Autodesk Fusion 360 part; units mm, degrees
sketch "Sketch1" plane through (0, 0, 0) normal (0, 1, 0) x (1, 0, 0)
  line L0 (0, 0) -> (60, 0)
  line L1 (60, 0) -> (-60, 0)
  line L2 (-60, 0) -> (-60, -50)
  line L3 (-60, -50) -> (60, -50)
  line L4 (60, -50) -> (60, 0)
  line L5 (-60, 0) -> (-45, 0)
  line L6 (60, 0) -> (45, 0)
  line L7 (-45, 0) -> (-45, 60)
  line L8 (45, 0) -> (45, 60)
  line L9 (-45, 60) -> (45, 60)
  dimension "d1" = 60
  dimension "d2" = 120
  dimension "d3" = 50
  dimension "d4" = 15
  dimension "d5" = 15
  dimension "d6" = 60
  dimension "d7" = 60
extrude "Extrude1" add sketch "Sketch1" along normal blind 10
sketch "Sketch2" plane through (0, 10, 0) normal (0, 1, 0) x (-1, 0, 0)
  line L0 (60, 0) -> (60, 50)
  line L1 (60, 50) -> (-60, 50)
  line L2 (-60, 50) -> (-60, 0)
  line L3 (-60, 0) -> (-45, 0)
  line L4 (-45, 0) -> (-45, -60)
  line L5 (-45, -60) -> (45, -60)
  line L6 (45, -60) -> (45, 0)
  line L7 (45, 0) -> (60, 0)
  line L8 (60, 50) -> (60, 40)
  line L9 (-60, 50) -> (-60, 40)
  circle A0 centre (50, 40) radius 2.5
  circle A1 centre (-50, 40) radius 2.5
  circle A2 centre (50, 10) radius 2.5
  circle A3 centre (-50, 10) radius 2.5
  dimension "d10" = 10
  dimension "d11" = 10
  dimension "d12" = 10
  dimension "d13" = 10
  dimension "d14" = 5
  dimension "d15" = 5
  dimension "d16" = 30
  dimension "d17" = 5
  dimension "d18" = 30
  dimension "d19" = 5
extrude "Extrude2" cut sketch "Sketch2" against normal blind 20 contours A0 | A1 | A2 | A3
sketch "Sketch3" plane through (0, 10, 0) normal (0, 1, 0) x (-1, 0, 0)
  circle A0 centre (50, 40) radius 2.5
  circle A1 centre (-50, 40) radius 2.5
  circle A2 centre (50, 10) radius 2.5
  circle A3 centre (-50, 10) radius 2.5
  line L0 (60, 0) -> (60, 50)
  line L1 (60, 50) -> (-60, 50)
  line L2 (-60, 50) -> (-60, 0)
  line L3 (-60, 0) -> (-45, 0)
  line L4 (-45, 0) -> (-45, -60)
  line L5 (-45, -60) -> (45, -60)
  line L6 (45, -60) -> (45, 0)
  line L7 (45, 0) -> (60, 0)
  line L8 (45, -60) -> (45, 50)
  line L9 (-45, -60) -> (-45, 50)
  line L10 (45, 50) -> (-45, 50)
  line L11 (-45, -60) -> (45, -60)
  line L12 (45, 50) -> (42, 50)
  line L13 (45, -60) -> (42, -60)
  line L14 (-45, -60) -> (-45, -57)
  line L15 (-45, 50) -> (-42, 50)
  line L16 (42, 47) -> (42, -57)
  line L17 (-42, -57) -> (42, -57)
  line L18 (-42, -57) -> (-42, 47)
  line L19 (-42, 47) -> (42, 47)
  dimension "d22" = 3
  dimension "d23" = 3
  dimension "d24" = 3
  dimension "d25" = 3
  dimension "d26" = 3
  dimension "d27" = 3
  dimension "d28" = 3
  dimension "d29" = 3
extrude "Extrude3" add sketch "Sketch3" along normal blind 70 contours L1 L4 L5 L6 L8 L9 L10 L11 L12 L13 L14 L15
sketch "Sketch4" plane through (-45, 0, 0) normal (-1, 0, 0) x (0, 0, 1)
  line L0 (-60, 0) -> (0, 0)
  line L1 (0, 0) -> (0, 10)
  line L2 (0, 10) -> (50, 10)
  line L3 (50, 10) -> (50, 80)
  line L4 (50, 80) -> (-60, 80)
  line L5 (-60, 80) -> (-60, 0)
  line L6 (-60, 80) -> (-60, 75)
  circle A0 centre (-35, 75) radius 2.5
  circle A1 centre (25, 75) radius 2.5
  dimension "d32" = 25
  dimension "d34" = 5
  dimension "d35" = 5
extrude "Extrude4" cut sketch "Sketch4" against normal blind 10 contours A0 | A1
sketch "Sketch5" plane through (45, 0, 0) normal (1, 0, 0) x (0, 0, -1)
  line L0 (0, 0) -> (60, 0)
  line L1 (60, 0) -> (60, 80)
  line L2 (60, 80) -> (-50, 80)
  line L3 (-50, 80) -> (-50, 10)
  line L4 (-50, 10) -> (0, 10)
  line L5 (0, 10) -> (0, 0)
  line L6 (-50, 80) -> (-50, 75)
  circle A0 centre (-25, 75) radius 2.5
  circle A1 centre (35, 75) radius 2.5
  dimension "d38" = 5
  dimension "d39" = 25
  dimension "d41" = 5
  dimension "d42" = 5
extrude "Extrude5" cut sketch "Sketch5" against normal blind 11 contours A0 | A1
sketch "Sketch6" plane through (0, 0, 50) normal (0, 0, 1) x (1, 0, 0)
  line L0 (-60, 0) -> (60, 0)
  line L1 (60, 0) -> (60, 10)
  line L2 (60, 10) -> (45, 10)
  line L3 (45, 10) -> (45, 80)
  line L4 (45, 80) -> (-45, 80)
  line L5 (-45, 80) -> (-45, 10)
  line L6 (-45, 10) -> (-60, 10)
  line L7 (-60, 10) -> (-60, 0)
  circle A0 centre (0, 75) radius 2.5
  dimension "d47" = 5
extrude "Extrude6" cut sketch "Sketch6" against normal blind 11 contours A0
sketch "Sketch7" plane through (0, 0, -60) normal (0, 0, -1) x (-1, 0, 0)
  line L0 (-45, 0) -> (45, 0)
  line L1 (45, 0) -> (45, 80)
  line L2 (45, 80) -> (-45, 80)
  line L3 (-45, 80) -> (-45, 0)
  circle A0 centre (0, 75) radius 2.5
  dimension "d51" = 5
extrude "Extrude7" cut sketch "Sketch7" against normal blind 11 contours A0
sketch "Sketch8" plane through (0, 0, 50) normal (0, 0, 1) x (1, 0, 0)
  circle A0 centre (0, 75) radius 2.5
  line L0 (-60, 0) -> (60, 0)
  line L1 (60, 0) -> (60, 10)
  line L2 (60, 10) -> (45, 10)
  line L3 (45, 10) -> (45, 80)
  line L4 (45, 80) -> (-45, 80)
  line L5 (-45, 80) -> (-45, 10)
  line L6 (-45, 10) -> (-60, 10)
  line L7 (-60, 10) -> (-60, 0)
  line L8 (-45, 80) -> (-45, 75)
  line L9 (-15, 77.5) -> (-35, 77.5)
  line L10 (-35, 72.5) -> (-15, 72.5)
  line L11 (-15, 77.5) -> (-10, 77.5)
  line L12 (-10, 77.5) -> (-10, 72.5)
  line L13 (-10, 72.5) -> (-15, 72.5)
  line L14 (-35, 77.5) -> (-40, 77.5)
  line L15 (-40, 77.5) -> (-40, 72.5)
  line L16 (-40, 72.5) -> (-35, 72.5)
  dimension "d55" = 20
  dimension "d56" = 5
  dimension "d57" = 5
extrude "Extrude8" cut sketch "Sketch8" against normal blind 20 contours L9 L10 L11 L12 L13 L14 L15 L16
sketch "Sketch9" plane through (0, 0, 50) normal (0, 0, 1) x (1, 0, 0)
  line L0 (-40, 72.5) -> (-40, 77.5)
  line L1 (-40, 77.5) -> (-10, 77.5)
  line L2 (-10, 77.5) -> (-10, 72.5)
  line L3 (-10, 72.5) -> (-40, 72.5)
  circle A0 centre (0, 75) radius 2.5
  line L4 (-60, 0) -> (60, 0)
  line L5 (60, 0) -> (60, 10)
  line L6 (60, 10) -> (45, 10)
  line L7 (45, 10) -> (45, 80)
  line L8 (45, 80) -> (-45, 80)
  line L9 (-45, 80) -> (-45, 10)
  line L10 (-45, 10) -> (-60, 10)
  line L11 (-60, 10) -> (-60, 0)
  line L12 (45, 80) -> (45, 75)
  line L13 (45, 75) -> (40, 75)
  line L14 (40, 75) -> (40, 72.5)
  line L15 (40, 75) -> (40, 77.5)
  line L16 (40, 77.5) -> (10, 77.5)
  line L17 (10, 77.5) -> (10, 72.5)
  line L18 (10, 72.5) -> (40, 72.5)
  dimension "d60" = 2.5
  dimension "d61" = 2.5
  dimension "d62" = 30
  dimension "d63" = 5
extrude "Extrude9" cut sketch "Sketch9" against normal blind 20 contours L14 L15 L16 L17 L18
sketch "Sketch10" plane through (0, 0, 0) normal (0, -1, 0) x (1, 0, 0)
  circle A0 centre (-50, 40) radius 2.5
  circle A1 centre (50, 40) radius 2.5
  circle A2 centre (-50, 10) radius 2.5
  circle A3 centre (50, 10) radius 2.5
  line L0 (-60, 50) -> (-60, 0)
  line L1 (-60, 0) -> (-45, 0)
  line L2 (-45, 0) -> (-45, -60)
  line L3 (-45, -60) -> (45, -60)
  line L4 (45, -60) -> (45, 0)
  line L5 (45, 0) -> (60, 0)
  line L6 (60, 0) -> (60, 50)
  line L7 (60, 50) -> (-60, 50)
  line L8 (0, 50) -> (11, 50)
  line L9 (11, 50) -> (11, 72)
  line L10 (11, 72) -> (-11, 72)
  line L11 (-11, 72) -> (-11, 50)
  line L12 (-11, 50) -> (-21, 50)
  line L13 (-21, 50) -> (-21, 80)
  line L14 (-21, 80) -> (21, 80)
  line L15 (21, 80) -> (21, 50)
  dimension "d66" = 11
  dimension "d67" = 22
  dimension "d68" = 22
  dimension "d69" = 10
extrude "Extrude10" add sketch "Sketch10" against normal blind 70 contours L7 L9 L10 L11 L12 L13 L14 L15
sketch "Sketch11" plane through (0, 0, 0) normal (0, -1, 0) x (1, 0, 0)
  line L0 (-21, 50) -> (-60, 50)
  line L1 (-60, 50) -> (-60, 0)
  line L2 (-60, 0) -> (-45, 0)
  line L3 (-45, 0) -> (-45, -60)
  line L4 (-45, -60) -> (45, -60)
  line L5 (45, -60) -> (45, 0)
  line L6 (45, 0) -> (60, 0)
  line L7 (60, 0) -> (60, 50)
  line L8 (60, 50) -> (21, 50)
  line L9 (21, 50) -> (21, 80)
  line L10 (21, 80) -> (-21, 80)
  line L11 (-21, 80) -> (-21, 50)
  circle A0 centre (-50, 40) radius 2.5
  circle A1 centre (50, 40) radius 2.5
  circle A2 centre (-50, 10) radius 2.5
  circle A3 centre (50, 10) radius 2.5
  line L12 (-11, 50) -> (-11, 72)
  line L13 (-11, 72) -> (11, 72)
  line L14 (11, 72) -> (11, 50)
  line L15 (11, 50) -> (-11, 50)
sketch "Sketch12" plane through (0, 0, 0) normal (0, -1, 0) x (1, 0, 0)
sketch "Sketch13" plane through (0, 0, 80) normal (0, 0, 1) x (1, 0, 0)
  line L0 (-21, 0) -> (21, 0)
  line L1 (21, 0) -> (21, 70)
  line L2 (21, 70) -> (-21, 70)
  line L3 (-21, 70) -> (-21, 0)
sketch "Sketch14" plane through (-45, 0, 0) normal (-1, 0, 0) x (0, 0, 1)
  circle A0 centre (25, 75) radius 2.5
  circle A1 centre (-35, 75) radius 2.5
  line L0 (-60, 0) -> (0, 0)
  line L1 (0, 0) -> (0, 10)
  line L2 (0, 10) -> (50, 10)
  line L3 (50, 10) -> (50, 80)
  line L4 (50, 80) -> (-60, 80)
  line L5 (-60, 80) -> (-60, 0)
  line L6 (0, 10) -> (25, 10)
  arc A2 (30, 10) -> (20, 10) centre (25, 10) ccw
  dimension "d72" = 10
extrude "Extrude11" cut sketch "Sketch14" against normal blind 100 contours L2 L6 A2
sketch "Sketch15" plane through (0, 0, -60) normal (0, 0, -1) x (-1, 0, 0)
  circle A0 centre (0, 75) radius 2.5
  line L0 (-45, 0) -> (45, 0)
  line L1 (45, 0) -> (45, 80)
  line L2 (45, 80) -> (-45, 80)
  line L3 (-45, 80) -> (-45, 0)
  line L4 (-45, 80) -> (-45, 65)
  line L5 (-30, 65) -> (-17, 65)
  line L6 (-30, 65) -> (-30, 47)
  line L7 (-30, 47) -> (-17, 47)
  line L8 (-17, 47) -> (-17, 65)
  dimension "d76" = 13
  dimension "d77" = 18
  dimension "d78" = 13
extrude "Extrude12" cut sketch "Sketch15" against normal blind 20 contours L5 L6 L7 L8
sketch "Sketch16" plane through (0, 0, -60) normal (0, 0, -1) x (-1, 0, 0)
  line L0 (-17, 47) -> (-30, 47)
  line L1 (-30, 47) -> (-30, 65)
  line L2 (-30, 65) -> (-17, 65)
  line L3 (-17, 65) -> (-17, 47)
  circle A0 centre (0, 75) radius 2.5
  line L4 (-45, 0) -> (45, 0)
  line L5 (45, 0) -> (45, 80)
  line L6 (45, 80) -> (-45, 80)
  line L7 (-45, 80) -> (-45, 0)
  line L8 (-5, 65) -> (5, 65)
  line L9 (-5, 65) -> (-5, 52)
  line L10 (-5, 52) -> (5, 52)
  line L11 (5, 52) -> (5, 65)
  dimension "d81" = 10
  dimension "d82" = 13
  dimension "d83" = 10
extrude "Extrude13" cut sketch "Sketch16" against normal blind 20 contours L8 L9 L10 L11
sketch "Sketch17" plane through (0, 80, 0) normal (0, 1, 0) x (-1, 0, 0)
  line L0 (42, -57) -> (-42, -57)
  line L1 (-42, -57) -> (-42, 47)
  line L2 (-42, 47) -> (42, 47)
  line L3 (42, 47) -> (42, -57)
  line L4 (-45, -60) -> (45, -60)
  line L5 (45, -60) -> (45, 50)
  line L6 (45, 50) -> (-45, 50)
  line L7 (-45, 50) -> (-45, -60)
sketch "Sketch18" plane through (0, 0, 50) normal (0, 0, 1) x (1, 0, 0)
  line L0 (-11, 70) -> (-11, 0)
  line L1 (-11, 0) -> (11, 0)
  line L2 (11, 0) -> (11, 70)
  line L3 (11, 70) -> (21, 70)
  line L4 (21, 70) -> (21, 0)
  line L5 (21, 0) -> (60, 0)
  line L6 (60, 0) -> (60, 10)
  line L7 (60, 10) -> (45, 10)
  line L8 (45, 10) -> (45, 80)
  line L9 (45, 80) -> (-45, 80)
  line L10 (-45, 80) -> (-45, 10)
  line L11 (-45, 10) -> (-60, 10)
  line L12 (-60, 10) -> (-60, 0)
  line L13 (-60, 0) -> (-21, 0)
  line L14 (-21, 0) -> (-21, 70)
  line L15 (-21, 70) -> (-11, 70)
  line L16 (10, 77.5) -> (40, 77.5)
  line L17 (40, 77.5) -> (40, 72.5)
  line L18 (40, 72.5) -> (10, 72.5)
  line L19 (10, 72.5) -> (10, 77.5)
  line L20 (-40, 72.5) -> (-40, 77.5)
  line L21 (-40, 77.5) -> (-10, 77.5)
  line L22 (-10, 77.5) -> (-10, 72.5)
  line L23 (-10, 72.5) -> (-40, 72.5)
  circle A0 centre (0, 75) radius 2.5
sketch "Sketch19" plane through (0, 80, 0) normal (0, 1, 0) x (-1, 0, 0)
sketch "Sketch20" plane through (0, 0, 50) normal (0, 0, 1) x (1, 0, 0)
sketch "Sketch21" plane through (-45, 0, 0) normal (-1, 0, 0) x (0, 0, 1)
  arc A0 (30, 10) -> (20, 10) centre (25, 10) ccw
  line L0 (30, 10) -> (50, 10)
  line L1 (50, 10) -> (50, 80)
  line L2 (50, 80) -> (-60, 80)
  line L3 (-60, 80) -> (-60, 0)
  line L4 (-60, 0) -> (0, 0)
  line L5 (0, 0) -> (0, 10)
  line L6 (0, 10) -> (20, 10)
  circle A1 centre (-35, 75) radius 2.5
  circle A2 centre (25, 75) radius 2.5
sketch "Sketch22" plane through (0, 80, 0) normal (0, 1, 0) x (-1, 0, 0)
sketch "Sketch23" plane through (-45, 0, 0) normal (-1, 0, 0) x (0, 0, 1)
sketch "Sketch24" plane through (45, 0, 0) normal (1, 0, 0) x (0, 0, -1)
  arc A0 (-20, 10) -> (-30, 10) centre (-25, 10) ccw
  line L0 (-20, 10) -> (0, 10)
  line L1 (0, 10) -> (0, 0)
  line L2 (0, 0) -> (60, 0)
  line L3 (60, 0) -> (60, 80)
  line L4 (60, 80) -> (-50, 80)
  line L5 (-50, 80) -> (-50, 10)
  line L6 (-50, 10) -> (-30, 10)
  circle A1 centre (35, 75) radius 2.5
  circle A2 centre (-25, 75) radius 2.5
sketch "Sketch25" plane through (0, 80, 0) normal (0, 1, 0) x (-1, 0, 0)
  point P0 (42, -57)
  point P1 (-42, -57)
  point P2 (42, 47)
  dimension "d86" = 84
  dimension "d87" = 104
The model under review builds one solid part; all positions refer to its coordinate system, in mm. A direction names the side the tool comes from. Give positions to 0.01 mm unless a question says otherwise; leave off trailing zeros. Write each loop counter-clockwise with the first axis right and the second up, starting at its lowest first coordinate (ties: lowest second). Pieces come first, ordered by that corner, then holes. Notation, with made-up numbers: M 64,53.25 L 84,53.25 A8 ccw 84,59.25 Z; hole C 34.5,-29.75 d8. An arc over 180 degrees is marked long. Answer in a Markdown table with one row per item.
Item 1: Draft analysis for pull direction X (two halves, no side actions). For faces 6 (the face through (0, 35, 72)), 7 (the face through (-43.52, 74.04, -32.69)), 8 (the face through (21, 35, 65)), 9 (the face through (-21, 35, 65)), state which applies: +X half, -X half, draft (parallel to the pull), parting line (faces both ways), or undercut.
Check sheet entries:
| item | result |
|---|---|
| face 6 | undercut |
| face 7 | draft |
| face 8 | +X half |
| face 9 | -X half |
Item 2: Add section A-A on x = 38. Give the boundary of the cut face in (y, z), plus the area to 4 significant figures.
Check sheet entries:
| item | result |
|---|---|
| outline | M 0,-60 L 80,-60 L 80,-57 L 10,-57 L 10,47 L 72.5,47 L 72.5,50 L 0,50 Z; M 77.5,47 L 80,47 L 80,50 L 77.5,50 Z |
| area | 1,505 mm2 |
Item 3: For line 1 along Z through (x, y) = (-50, 3.25); line 2 along Y through (x, z) = (-43.95, -35); line 3 along Z through (x, y) = (3.5, 42.5), list the stretches that pass through material, from the lowest coordinate up.
Check sheet entries:
| item | result |
|---|---|
| line 1 | 0 to 7.5, 12.5 to 37.5, 42.5 to 50 |
| line 2 | 0 to 72.5, 77.5 to 80 |
| line 3 | -60 to -57, 47 to 50, 72 to 80 |
Item 4: Add section D-D on y = 21.5. Give the boundary of the cut face in (x, z).
Check sheet entries:
| item | result |
|---|---|
| outline | M -45,-60 L 45,-60 L 45,50 L 21,50 L 21,80 L -21,80 L -21,50 L -45,50 Z; hole M -42,-57 L 42,-57 L 42,47 L -42,47 Z; hole M -11,50 L 11,50 L 11,72 L -11,72 Z |
Item 5: Add section B-B on x = -50. Give the boundary of the cut face in (y, z), plus the area to 3 significant figures.
Check sheet entries:
| item | result |
|---|---|
| outline | M 0,0 L 10,0 L 10,7.5 L 0,7.5 Z; M 0,12.5 L 10,12.5 L 10,37.5 L 0,37.5 Z; M 0,42.5 L 10,42.5 L 10,50 L 0,50 Z |
| area | 400 mm2 |
Item 6: For P1, Ø2.5, axis at y = 57.5, z = -58.5, coming from the +X side; P2, Ø2.5, axis at y = 74.5, z = 48.5, coming from the -X side; P3, Ø8, axis at x = -50, y = 4.5, coming from the -Z side, all flat-tipped, find the tip position at first contact; note any pin that passes through.
Check sheet entries:
| item | result |
|---|---|
| P1 | x = 45 |
| P2 | x = -45 |
| P3 | z = 0 |
Item 7: Add section C-C on z = 68. Give the boundary of the cut face in (x, y).
Check sheet entries:
| item | result |
|---|---|
| outline | M -21,0 L -11,0 L -11,70 L -21,70 Z; M 11,0 L 21,0 L 21,70 L 11,70 Z |
Item 8: Tool access review of faces 1 (the face through (-0.54, 72.56, 48.52)), 2 (the face through (0, 70, 75)), 3 (the face through (1, 45, -57)), 4 (the face through (-44, 15, 25)), 5 (the face through (-11, 35, 61)): name each direction out of +Z, -Z, +X, -X, +Y, -Y from which nothing blocks a thin tool from reaching the whole face with its end or side.
Check sheet entries:
| item | result |
|---|---|
| face 1 | +Z, -Z |
| face 2 | +Z, +X, -X, +Y |
| face 3 | +Y |
| face 4 | +X, -X |
| face 5 | +Y, -Y |
